Can you work these out from the model? Positions are in its coordinate system, mm. Face numbers are marked on the shaded views. A direction names the side the tool comes from. Give positions to 0.01 mm unless a question says otherwise; leave off trailing zeros. Order: outer loops, then holes, each group sorted by start corner. A loop starts at its lowest first (then second) coordinate and runs counter-clockwise, first axis right, second up. Notation, with made-up numbers: (10, 42) - (68, 42) arc R29 ccw to (68, 72) - close; hole circle Ø7 at (-12, 72.25). An arc over 180 degrees is marked (long way). Answer as CSV lines item,"result".
```python
from build123d import *

# Parameters (mm, degrees)
SKETCH1_W           = 100
SKETCH1_H           = 100
BOSS_EXTRUDE1_DEPTH = 4.5
SKETCH2_W           = 3
SKETCH2_H           = 15
BOSS_EXTRUDE2_DEPTH = 60
SKETCH3_R           = 4
CUT_EXTRUDE1_DEPTH  = 96
SKETCH4_R           = 1.5
BOSS_EXTRUDE3_DEPTH = 3


with BuildPart() as part:
    # Sketch1 → Boss-Extrude1 (new body)
    with BuildSketch(Plane(origin=(0, 0, 0), x_dir=(1, 0, 0), z_dir=(0, 1, 0))):
        Rectangle(SKETCH1_W, SKETCH1_H)
    extrude(amount=BOSS_EXTRUDE1_DEPTH)

    # Sketch2 → Boss-Extrude2 (add)
    with BuildSketch(Plane(origin=(0, 4.5, 0), x_dir=(1, 0, 0), z_dir=(0, 1, 0))):
        with Locations((43.5, 0)):
            Rectangle(SKETCH2_W, SKETCH2_H)
        with Locations((-43.5, 0)):
            Rectangle(SKETCH2_W, SKETCH2_H)
    extrude(amount=BOSS_EXTRUDE2_DEPTH)

    # Sketch3 → Cut-Extrude1 (cut, through all)
    with BuildSketch(Plane(origin=(45, 0, 0), x_dir=(0, 0, -1), z_dir=(1, 0, 0))):
        with Locations((0, 54.5)):
            Circle(SKETCH3_R)
        with BuildLine():
            Line((-7.5, 54.5), (-7.5, 64.5))
            Line((-7.5, 64.5), (7.5, 64.5))
            Line((7.5, 64.5), (7.5, 54.5))
            ThreePointArc((7.5, 54.5), (0, 62), (-7.5, 54.5))
        make_face()
    extrude(amount=-CUT_EXTRUDE1_DEPTH, mode=Mode.SUBTRACT)

    # Sketch4 → Boss-Extrude3 (add)
    with BuildSketch(Plane(origin=(45, 0, 0), x_dir=(0, 0, -1), z_dir=(1, 0, 0))):
        Polygon((0, 27.02), (18.5, 27.02), (18.5, 37.02), (-18.5, 37.02), (-18.5, 27.02), align=None)
        with Locations((-10, 32.02)):
            Circle(SKETCH4_R, mode=Mode.SUBTRACT)
        with Locations((10, 32.02)):
            Circle(SKETCH4_R, mode=Mode.SUBTRACT)
    extrude(amount=-BOSS_EXTRUDE3_DEPTH)


solid = part.part
```
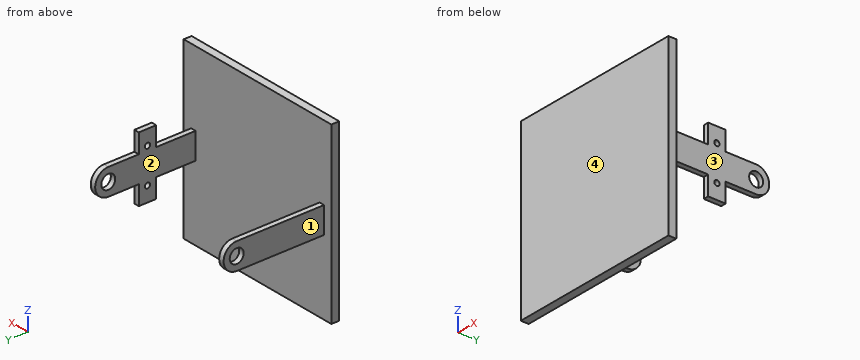
1) I want a section at C-C on y = 14. Write out the boundary of the cut face in (x, z), plus the area to 3 significant figures.
Answer block:
outline,"(-45, -7.5) - (-42, -7.5) - (-42, 7.5) - (-45, 7.5) - close; (42, -7.5) - (45, -7.5) - (45, 7.5) - (42, 7.5) - close"
area,"90.0 mm2"
2) I need wall thicknesses on line 1 along Y through (x, z) = (44.1, 10); line 2 along X through (y, z) = (5.5, 5.5); line 3 along Z through (x, y) = (43, 54). Which ranges of each line are inside material? Lowest first, please. Write a range as [from, to].
Answer block:
line 1,"[0, 4.5], [27.02, 30.52], [33.52, 37.02]"
line 2,"[-45, -42], [42, 45]"
line 3,"[-7.5, -3.97], [3.97, 7.5]"
3) I want a section at A-A on z = 0. Write out the boundary of the cut face in (x, y), plus the area to 3 significant figures.
Answer block:
outline,"(-50, 0) - (50, 0) - (50, 4.5) - (45, 4.5) - (45, 50.5) - (42, 50.5) - (42, 4.5) - (-42, 4.5) - (-42, 50.5) - (-45, 50.5) - (-45, 4.5) - (-50, 4.5) - close; (-45, 58.5) - (-42, 58.5) - (-42, 62) - (-45, 62) - close; (42, 58.5) - (45, 58.5) - (45, 62) - (42, 62) - close"
area,"747 mm2"
4) I want a section at B-B on y = 32.02. Write out the boundary of the cut face in (x, z).
Answer block:
outline,"(-45, -7.5) - (-42, -7.5) - (-42, 7.5) - (-45, 7.5) - close; (42, -18.5) - (45, -18.5) - (45, -11.5) - (42, -11.5) - close; (42, -8.5) - (45, -8.5) - (45, 8.5) - (42, 8.5) - close; (42, 11.5) - (45, 11.5) - (45, 18.5) - (42, 18.5) - close"
5) Which directions (+Z, -Z, +X, -X, +Y, -Y) give clear straight access to the entire face, cutting with the end or side of a thin tool? Please do the marked faces 1, 2, 3 and 4.
Answer block:
face 1,"+Z, -Z, -X, +Y"
face 2,"+Z, -Z, +Y"
face 3,"+Z, -Z, +X, +Y"
face 4,"+Z, -Z, +X, -X, -Y"
6) I'm going to push flat-ended pins straight in: P1, Ø4.5, axis at y = 41, z = 3, coming from the -X side; P2, Ø16.5, axis at y = 47.5, z = -1, coming from the +X side; P3, Ø0.9, axis at x = 43, z = -11.5, coming from the +Y side; P4, Ø12, axis at y = 42.5, z = 28.5, coming from the +X side. Where does each tip first touch, or does it pass through?
Answer block:
P1,"x = -45"
P2,"x = 45"
P3,"y = 37.02"
P4,"through"
7) I want a section at D-D on z = 10. Write out the boundary of the cut face in (x, y), plus the area to 3 significant figures.
Answer block:
outline,"(-50, 0) - (50, 0) - (50, 4.5) - (-50, 4.5) - close; (42, 27.02) - (45, 27.02) - (45, 30.52) - (42, 30.52) - close; (42, 33.52) - (45, 33.52) - (45, 37.02) - (42, 37.02) - close"
area,"471 mm2"
